```python
from build123d import *

# Parameters (mm, degrees)
F0_W     = 44.45
F0_H     = 76.2
F1_DEPTH = 57.15
F2_W     = 31.75
F2_H     = 25.4
F3_DEPTH = 3.175
F4_W     = 31.75
F4_H     = 25.4
F5_DEPTH = 3.175


with BuildPart() as f1:
    # F0 (on Right) → F1 (new body)
    with BuildSketch(Plane.YZ):
        with Locations((22.225, -38.1)):
            Rectangle(F0_W, F0_H)
    extrude(amount=F1_DEPTH)

    # F2 (on face) → F3 (cut)
    with BuildSketch(Plane.YZ.offset(57.15)):
        with Locations((22.225, -19.05)):
            Rectangle(F2_W, F2_H)
    extrude(amount=-F3_DEPTH, mode=Mode.SUBTRACT)

    # F4 (on face) → F5 (cut)
    with BuildSketch(Plane(origin=(0, 0, 0), x_dir=(0, -1, 0), z_dir=(-1, 0, 0))):
        with Locations((-22.225, -19.05)):
            Rectangle(F4_W, F4_H)
    extrude(amount=-F5_DEPTH, mode=Mode.SUBTRACT)


solid = f1.part
```
The model under review builds one solid part; all positions refer to its coordinate system, in mm. A direction names the side the tool comes from. Round coordinates to 2 decimals unless told otherwise and drop trailing zeros. Order: outer loops, then holes, each group sorted by start corner. A loop starts at its lowest first (then second) coordinate and runs counter-clockwise, first axis right, second up. Notation, with made-up numbers: M 46,52 L 70,52 A25 cw 70,66 Z; hole C 40,-8.5 d3. An arc over 180 degrees is marked long. Use a Markdown table: item, result.
1) Tool access review of faces 1 (the face through (57.15, 22, -46)), 2 (the face through (2, 22, -31.75)), 3 (the face through (56, 22, -6.35)): name each direction out of +Z, -Z, +X, -X, +Y, -Y from which nothing blocks a thin tool from reaching the whole face with its end or side.
Report:
| item | result |
|---|---|
| face 1 | +Z, -Z, +X, +Y, -Y |
| face 2 | -X |
| face 3 | +X |
2) Wall thickness on line 1 along Y through (x, z) = (55, -8.5); line 2 along X through (y, z) = (27.5, -17.5) (3 decimals): over which ranges is each line inside the solid? List them lowest first. Write a range as [from, to].
Report:
| item | result |
|---|---|
| line 1 | [0, 6.35], [38.1, 44.45] |
| line 2 | [3.175, 53.975] |
3) Draft analysis for pull direction Z (two halves, no side actions). For faces 4 (the face through (53.975, 22, -19)), 5 (the face through (28, 22, 0)), 6 (the face through (28, 0, -39)), state which applies: released by +Z, released by -Z, zero draft, split by the parting line, or undercut.
Report:
| item | result |
|---|---|
| face 4 | undercut |
| face 5 | released by +Z |
| face 6 | zero draft |
4) Consider section B-B (y = 12.5). Write out the cut boundary in (x, z) (3 decimals), then the cut area to 3 significant figures.
Report:
| item | result |
|---|---|
| outline | M 0,-76.2 L 57.15,-76.2 L 57.15,-31.75 L 53.975,-31.75 L 53.975,-6.35 L 57.15,-6.35 L 57.15,0 L 0,0 L 0,-6.35 L 3.175,-6.35 L 3.175,-31.75 L 0,-31.75 Z |
| area | 4,190 mm^2 |
5) Consider section A-A (z = -16.5). Write out the cut boundary in (x, y) (3 decimals), then the cut area to 3 significant figures.
Report:
| item | result |
|---|---|
| outline | M 0,0 L 57.15,0 L 57.15,6.35 L 53.975,6.35 L 53.975,38.1 L 57.15,38.1 L 57.15,44.45 L 0,44.45 L 0,38.1 L 3.175,38.1 L 3.175,6.35 L 0,6.35 Z |
| area | 2,340 mm^2 |
